Autodesk Inventor part; units mm, degrees
ref_plane "YZ Plane" through (0, 0, 0) normal (1, 0, 0) x (0, 1, 0)
ref_plane "XZ Plane" through (0, 0, 0) normal (0, 1, 0) x (-1, 0, 0)
ref_plane "XY Plane" through (0, 0, 0) normal (0, 0, 1) x (1, 0, 0)
ref_plane "Work Plane1" through (0, 0, 0) normal (0, 0, 1) x (1, 0, 0)
sketch "Sketch1" plane through (0, 0, 0) normal (0, 0, 1) x (1, 0, 0)
  line L0 (26.085, -12.7501) -> (26.085, -38.7501)
  line L1 (15.085, -12.7501) -> (26.085, -12.7501)
  line L2 (15.085, -38.7501) -> (15.085, -12.7501)
  line L3 (26.085, -38.7501) -> (15.085, -38.7501)
  line L4 (26.085, -25.7501) -> (15.085, -25.7501)
  line L5 (20.585, -38.7501) -> (20.585, -12.7501)
  line L6 (15.2194, -38.2641) -> (25.9506, -38.2641)
  line L7 (25.9506, -38.2641) -> (25.9506, -13.236)
  line L8 (25.9506, -13.236) -> (15.2194, -13.236)
  line L9 (15.2194, -13.236) -> (15.2194, -38.2641)
  line L10 (15.2194, -38.2641) -> (25.9506, -13.236) construction
  line L11 (25.9506, -38.2641) -> (15.2194, -13.236) construction
  point P0 (0, 0)
  point P1 (20.585, -25.7501)
extrude "Extrusion1" add sketch "Sketch1" against normal blind 1 contours L7 L6 L5 L4 | L4 L5 L8 L7 | L5 L4 L9 L8 | L5 L6 L9 L4
sketch "Sketch2" plane through (0, 0, 0) normal (0, 0, 1) x (1, 0, 0)
  line L0 (15.2194, -13.236) -> (15.2194, -38.2641)
  line L1 (15.2194, -38.2641) -> (25.9506, -38.2641)
  line L2 (25.9506, -38.2641) -> (25.9506, -13.236)
  line L3 (25.9506, -13.236) -> (15.2194, -13.236)
  line L4 (13.1635, -39.268) -> (28.9935, -39.268)
  line L5 (28.9935, -39.268) -> (28.9935, -12.2321)
  line L6 (28.9935, -12.2321) -> (13.1635, -12.2321)
  line L7 (13.1635, -12.2321) -> (13.1635, -39.268)
  line L8 (13.1635, -39.268) -> (28.9935, -12.2321) construction
  line L9 (28.9935, -39.268) -> (13.1635, -12.2321) construction
  line L10 (28.9935, -12.2321) -> (32.8035, -12.2321)
  line L11 (32.8035, -12.2321) -> (32.8035, -16.0421)
  line L12 (32.8035, -16.0421) -> (28.9935, -16.0421)
  line L13 (28.9935, -39.268) -> (32.8035, -39.268)
  line L14 (32.8035, -39.268) -> (32.8035, -35.458)
  line L15 (32.8035, -35.458) -> (28.9935, -35.458)
  line L16 (13.1635, -12.2321) -> (3.8747, -12.2321)
  line L17 (3.8747, -12.2321) -> (3.8747, -16.0421)
  line L18 (3.8747, -16.0421) -> (13.1635, -16.0421)
  line L19 (13.1635, -39.268) -> (3.8747, -39.268)
  line L20 (3.8747, -39.268) -> (3.8747, -35.458)
  line L21 (3.8747, -35.458) -> (13.1635, -35.458)
  circle A0 centre (30.455, -14.1001) radius 1
  circle A1 centre (30.455, -37.4001) radius 1
  circle A2 centre (6.655, -37.4001) radius 1
  circle A3 centre (6.655, -14.1001) radius 1
  point P0 (0, 0)
  point P1 (21.0785, -25.7501)
  dimension "d2" = 3.81
  dimension "d3" = 3.81
  dimension "d4" = 3.81
  dimension "d5" = 3.81
  dimension "d6" = 6.0858
  dimension "d7" = 4.1119
  dimension "d8" = 27.0359
  dimension "d9" = 3.81
  dimension "d10" = 3.81
  dimension "d11" = 2.0078
  dimension "d12" = 44.1517
extrude "Extrusion2" add sketch "Sketch2" along normal blind 3 contours L3 L2 L1 L0 | L7 L6 L5 L4 | L19 L20 L21 L7 | L5 L15 L14 L13 | L18 L17 L16 L7 | L5 L10 L11 L12
fillet "Fillet1" radius 0.3175 30 edges at (32.8035, -16.0421, 1.5) (32.8035, -12.2321, 1.5) (30.8985, -16.0421, 3) (18.3391, -12.2321, 3) (28.9935, -25.7501, 3) (28.9935, -16.0421, 1.5) (30.8985, -16.0421, 0) (28.9935, -25.7501, 0) (32.8035, -35.458, 1.5) (30.8985, -35.458, 3) (18.3391, -39.268, 3) (32.8035, -39.268, 1.5) (32.8035, -37.363, 3) (32.8035, -14.1371, 3) (28.9935, -35.458, 1.5) (30.8985, -35.458, 0) (18.3391, -39.268, 0) (3.8747, -39.268, 1.5) (3.8747, -37.363, 3) (8.5191, -35.458, 3) (13.1635, -25.7501, 3) (8.5191, -16.0421, 3) (3.8747, -16.0421, 1.5) (3.8747, -14.1371, 3) (18.3391, -12.2321, 0) (3.8747, -12.2321, 1.5) (8.5191, -16.0421, 0) (8.5191, -35.458, 0) (32.8035, -37.363, 0) (32.8035, -14.1371, 0)
properties part number "OLED"
Geometry check sheet. Reference: the model listing, model coordinates, mm. A direction names the side the tool comes from. Coordinates: 2 decimals unless noted, no trailing zeros. Order: outer loops, then holes, each group sorted by start corner. A loop starts at its lowest first (then second) coordinate and runs counter-clockwise, first axis right, second up. Notation, with made-up numbers: (54.5, 18.25) - (100.5, 18.25) arc R16 cw to (100.5, 23.25) - close; hole circle Ø2 at (46, 42). An arc over 180 degrees is marked (long way). Answer in a Markdown table with one row per item. Add a question column.
1) Material ranges on line 1 along X through (y, z) = (-37.5, 1.5); line 2 along Y through (x, z) = (30.75, 0.9); line 3 along Y through (x, z) = (30, 0.25), recorded low to high. Write a range as [from, to].
2) Cross-section at D-D, the plane x = 23.5. Record the cut outline in (y, z) (1 decimal), then the cut area to 3 significant figures.
3) Cross-section at A-A, the plane x = 8.25. Record the cut outline in (y, z) (1 decimal), then the cut area to 3 significant figures.
4) Gauge pin test, flat ends, axial feed: P1, Ø0.8, axis at x = 20.5, z = -0.5, coming from the -Y side; P2, Ø1.5, axis at y = -31.5, z = 2.5, coming from the +X side; P3, Ø1.1, axis at y = -21.5, z = -0.5, coming from the -X side; P4, Ø1.6, axis at x = 6.66, y = -37.4, coming from the +Z side. Record the tip position at first contact, or that the pin passes through.
5) Release check for a two-part mould opening along Y. For faces 5 (the cylindrical face through (29.456, -37.444, 1.479)), 6 (the flat face through (32.804, -37, 1)), 7 (the flat face through (20.5, -38.264, -0.5)), 8 (the cylindrical face through (6.438, -36.424, 1.479)) record: +Y half, -Y half, draft (parallel to the pull), parting line (faces both ways), or undercut.
6) Cross-section at C-C, the plane y = -22. Record the cut outline in (x, z) (1 decimal), then the cut area to 3 significant figures.
7) Set-up check for faces 1 (the flat face through (28.994, -26, 1)), 2 (the flat face through (20.7, -13.236, -0.5)), 3 (the flat face through (25.951, -25.9, -0.5)), 4 (the flat face through (9, -16.042, 1)): record each of +Z, -Z, +X, -X, +Y, -Y from which the full face is reachable in a straight line by a thin tool's end or side.
8) Cross-section at B-B, the plane z = 1.7. Record the cut outline in (x, y) (1 decimal).
Check result:
| question | item | result |
|---|---|---|
| 1 | line 1 | x = [3.87, 5.66], [7.65, 29.46], [31.45, 32.8] |
| 1 | line 2 | y = [-39.27, -38.36], [-36.44, -35.46], [-16.04, -15.06], [-13.14, -12.23] |
| 1 | line 3 | y = [-39.26, -38.29], [-36.51, -35.47], [-16.03, -14.99], [-13.21, -12.24] |
| 2 | outline | (-39.3, 0.3) arc R0.3 ccw to (-39, 0) - (-38.3, 0) - (-38.3, -1) - (-13.2, -1) - (-13.2, 0) - (-12.5, 0) arc R0.3 ccw to (-12.2, 0.3) - (-12.2, 2.7) arc R0.3 ccw to (-12.5, 3) - (-39, 3) arc R0.3 ccw to (-39.3, 2.7) - close |
| 2 | area | 106 mm² |
| 3 | outline | (-39.3, 0.3) arc R0.3 ccw to (-39, 0) - (-35.8, 0) arc R0.3 ccw to (-35.5, 0.3) - (-35.5, 2.7) arc R0.3 ccw to (-35.8, 3) - (-39, 3) arc R0.3 ccw to (-39.3, 2.7) - close; (-16, 0.3) arc R0.3 ccw to (-15.7, 0) - (-12.5, 0) arc R0.3 ccw to (-12.2, 0.3) - (-12.2, 2.7) arc R0.3 ccw to (-12.5, 3) - (-15.7, 3) arc R0.3 ccw to (-16, 2.7) - close |
| 3 | area | 22.7 mm² |
| 4 | P1 | stops at y = -38.26 |
| 4 | P2 | stops at x = 28.99 |
| 4 | P3 | stops at x = 13.16 |
| 4 | P4 | passes through |
| 5 | face 5 | undercut |
| 5 | face 6 | draft |
| 5 | face 7 | -Y half |
| 5 | face 8 | undercut |
| 6 | outline | (13.2, 0) - (15.2, 0) - (15.2, -1) - (26, -1) - (26, 0) - (28.7, 0) arc R0.3 ccw to (29, 0.3) - (29, 2.7) arc R0.3 ccw to (28.7, 3) - (13.5, 3) arc R0.3 ccw to (13.2, 2.7) - close |
| 6 | area | 58.2 mm² |
| 7 | face 1 | +Z, -Z, +X |
| 7 | face 2 | -Z, +X, -X, +Y |
| 7 | face 3 | -Z, +X, +Y, -Y |
| 7 | face 4 | +Z, -Z, -X |
| 8 | outline | (3.9, -39) arc R0.3 ccw to (4.2, -39.3) - (32.5, -39.3) arc R0.3 ccw to (32.8, -39) - (32.8, -35.8) arc R0.3 ccw to (32.5, -35.5) - (29.3, -35.5) arc R0.3 cw to (29, -35.1) - (29, -16.4) arc R0.3 cw to (29.3, -16) - (32.5, -16) arc R0.3 ccw to (32.8, -15.7) - (32.8, -12.5) arc R0.3 ccw to (32.5, -12.2) - (4.2, -12.2) arc R0.3 ccw to (3.9, -12.5) - (3.9, -15.7) arc R0.3 ccw to (4.2, -16) - (13.2, -16) - (13.2, -35.5) - (3.9, -35.5) - close; hole circle Ø2 at (6.7, -37.4); hole circle Ø2 at (6.7, -14.1); hole circle Ø2 at (30.5, -37.4); hole circle Ø2 at (30.5, -14.1) |
